Input: dimensioned drawing with shaded views. Units: mm. Origin: part minimum x, y, z. Round coordinates to 2 decimals unless told otherwise and drop trailing zeros. Order: outer loops, then holes, each group sorted by start corner. A loop starts at its lowest first (then second) coordinate and runs counter-clockwise, first axis right, second up. Notation, with made-up numbers: M -4,2 L 19,2 A28 ccw 19,35 Z; hole C 36.25,38 d1. An arc over 180 degrees is marked long. Answer as CSV lines item,"result". Start each with the question number.
Item 1: First-contact query: P1, Ø15.5, axis at x = 345, z = 25, coming from the -Y side; P2, Ø3, axis at x = 136.5, z = 180, coming from the -Y side. Flat tips, straight axial feed; report the tip coordinate or a pass-through.
Item 2: Line query: line 1 (Z direction, x = 20, y = 6); line 2 (X direction, y = 9.5, z = 247); line 3 (X direction, y = 4.5, z = 91.5). Output: solid intervals per line, ascending. Write a range as [from, to].
Item 3: Section query B-B on z = 180.5. Return the cut outline in (x, y), plus the area to 3 significant figures.
Item 4: Section query A-A on x = 345. Return the cut outline in (y, z), plus the area to 3 significant figures.
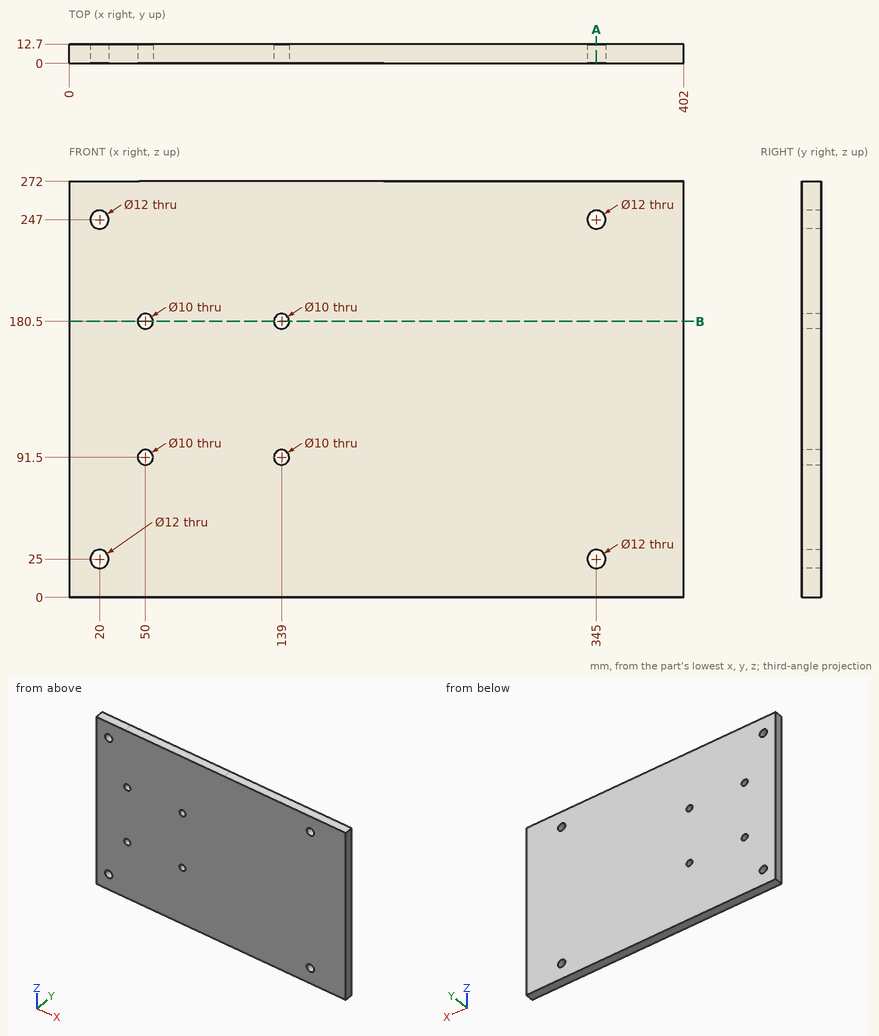
Results:
1,P1,"y = 0"
1,P2,"through"
2,line 1,"[0, 19], [31, 241], [253, 272]"
2,line 2,"[0, 14], [26, 339], [351, 402]"
2,line 3,"[0, 45], [55, 134], [144, 402]"
3,outline,"M 0,0 L 45,0 L 45,12.7 L 0,12.7 Z; M 55,0 L 134,0 L 134,12.7 L 55,12.7 Z; M 144,0 L 402,0 L 402,12.7 L 144,12.7 Z"
3,area,"4,850 mm^2"
4,outline,"M 0,0 L 12.7,0 L 12.7,19 L 0,19 Z; M 0,31 L 12.7,31 L 12.7,241 L 0,241 Z; M 0,253 L 12.7,253 L 12.7,272 L 0,272 Z"
4,area,"3,150 mm^2"
